Could you check a few things on this model? Use its own coordinates, in mm. Face numbers are marked on the shaded views. A direction names the side the tool comes from. Give positions to 0.01 mm unless a question says otherwise; leave off trailing zeros. Write each loop counter-clockwise with the first axis right and the second up, starting at its lowest first coordinate (ties: lowest second). Pieces come first, ordered by that corner, then holes. Notation, with made-up numbers: (-13.75, 63) - (1.25, 63) arc R20 cw to (1.25, 98) - close; hole circle Ø7 at (87, 20.25). An arc over 180 degrees is marked (long way). Use one line per item in the form item = value.
```python
from build123d import *

# Parameters (mm, degrees)
SKETCH1_W           = 40
SKETCH1_H           = 24
BOSS_EXTRUDE1_DEPTH = 1
SKETCH2_W           = 40
SKETCH2_H           = 24
SKETCH2_W_2         = 21
SKETCH2_H_2         = 17.5
SKETCH2_W_3         = 13
SKETCH2_H_3         = 18.5
BOSS_EXTRUDE3_DEPTH = 8
SKETCH3_W           = 1
SKETCH3_H           = 17.5
CUT_EXTRUDE2_DEPTH  = 3
SKETCH4_W           = 10.24
SKETCH4_H           = 11.92
BOSS_EXTRUDE4_DEPTH = 1.21
CUT_EXTRUDE3_DEPTH  = 2
SKETCH8_W           = 4
SKETCH8_H           = 18.5
CUT_EXTRUDE4_DEPTH  = 5
SKETCH11_W          = 24
SKETCH11_H          = 9
CUT_EXTRUDE5_DEPTH  = 2
SKETCH12_W          = 4
SKETCH12_H          = 3
CUT_EXTRUDE6_DEPTH  = 3
BOSS_EXTRUDE5_DEPTH = 3.5
SKETCH14_W          = 1
SKETCH14_H          = 2.25
CUT_EXTRUDE7_DEPTH  = 3


with BuildPart() as part:
    # Sketch1 → Boss-Extrude1 (new body)
    with BuildSketch(Plane(origin=(0, 0, 0), x_dir=(1, 0, 0), z_dir=(0, 1, 0))):
        with Locations((20, 12)):
            Rectangle(SKETCH1_W, SKETCH1_H)
    extrude(amount=BOSS_EXTRUDE1_DEPTH)

    # Sketch2 → Boss-Extrude3 (add)
    with BuildSketch(Plane(origin=(0, 1, 0), x_dir=(1, 0, 0), z_dir=(0, 1, 0))):
        with Locations((20, 12)):
            Rectangle(SKETCH2_W, SKETCH2_H)
        with Locations((11.5, 12)):
            Rectangle(SKETCH2_W_2, SKETCH2_H_2, mode=Mode.SUBTRACT)
        with Locations((29.5, 12)):
            Rectangle(SKETCH2_W_3, SKETCH2_H_3, mode=Mode.SUBTRACT)
    extrude(amount=BOSS_EXTRUDE3_DEPTH)

    # Sketch3 → Cut-Extrude2 (cut)
    with BuildSketch(Plane(origin=(0, 9, 0), x_dir=(1, 0, 0), z_dir=(0, 1, 0))):
        with Locations((22.5, 12)):
            Rectangle(SKETCH3_W, SKETCH3_H)
    extrude(amount=-CUT_EXTRUDE2_DEPTH, mode=Mode.SUBTRACT)

    # Sketch4 → Boss-Extrude4 (add)
    with BuildSketch(Plane(origin=(0, 1, 0), x_dir=(1, 0, 0), z_dir=(0, 1, 0))):
        with Locations((13.26, 12)):
            Rectangle(SKETCH4_W, SKETCH4_H)
    extrude(amount=BOSS_EXTRUDE4_DEPTH)

    # Sketch5 → Cut-Extrude3 (cut)
    with BuildSketch(Plane(origin=(1, 0, 0), x_dir=(0, 0, -1), z_dir=(1, 0, 0))):
        with BuildLine():
            Line((7.53, 2.25), (7.53, 2.96))
            Line((7.53, 2.96), (7.53, 9))
            Line((7.53, 9), (16.47, 9))
            Line((16.47, 9), (16.47, 2.96))
            Line((16.47, 2.96), (16.47, 2.25))
            ThreePointArc((16.47, 2.25), (16.103883476, 1.366116524), (15.22, 1))
            Line((15.22, 1), (8.78, 1))
            ThreePointArc((8.78, 1), (7.896116524, 1.366116524), (7.53, 2.25))
        make_face()
    extrude(amount=-CUT_EXTRUDE3_DEPTH, mode=Mode.SUBTRACT)

    # Sketch8 → Cut-Extrude4 (cut)
    with BuildSketch(Plane(origin=(0, 9, 0), x_dir=(1, 0, 0), z_dir=(0, 1, 0))):
        with Locations((38, 12)):
            Rectangle(SKETCH8_W, SKETCH8_H)
    extrude(amount=-CUT_EXTRUDE4_DEPTH, mode=Mode.SUBTRACT)

    # Sketch11 → Cut-Extrude5 (cut)
    with BuildSketch(Plane(origin=(40, 0, 0), x_dir=(0, 0, -1), z_dir=(1, 0, 0))):
        with Locations((12, 4.5)):
            Rectangle(SKETCH11_W, SKETCH11_H)
    extrude(amount=-CUT_EXTRUDE5_DEPTH, mode=Mode.SUBTRACT)

    # Sketch12 → Cut-Extrude6 (cut)
    with BuildSketch(Plane(origin=(0, 9, 0), x_dir=(1, 0, 0), z_dir=(0, 1, 0))):
        with Locations((6, 2.5)):
            Rectangle(SKETCH12_W, SKETCH12_H)
    extrude(amount=-CUT_EXTRUDE6_DEPTH, mode=Mode.SUBTRACT)

    # Sketch13 → Boss-Extrude5 (add)
    with BuildSketch(Plane(origin=(0, 9, 0), x_dir=(1, 0, 0), z_dir=(0, 1, 0))):
        Polygon((1, 16.47), (1, 20.75), (3, 20.75), (3, 15.25), (1, 15.25), (1, 16.25), (0, 16.25), (0, 16.47), align=None)
        Polygon((1, 3.25), (3, 3.25), (3, 8.75), (1, 8.75), (1, 7.75), (0, 7.75), (0, 7.53), (1, 7.53), align=None)
    extrude(amount=-BOSS_EXTRUDE5_DEPTH)

    # Sketch14 → Cut-Extrude7 (cut)
    with BuildSketch(Plane(origin=(0, 9, 0), x_dir=(1, 0, 0), z_dir=(0, 1, 0))):
        with Locations((3.5, 2.125)):
            Rectangle(SKETCH14_W, SKETCH14_H)
    extrude(amount=-CUT_EXTRUDE7_DEPTH, mode=Mode.SUBTRACT)


solid = part.part
```
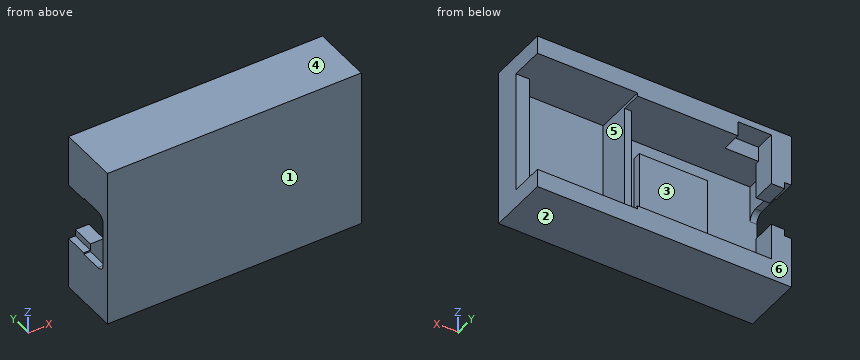
1. Imagine slicing it at C-C, the plane z = -19.25. List the corners of the cut face in (x, y) for me, and give its area (3 significant figures).
Response values:
outline = (0, 0) - (38, 0) - (38, 4) - (36, 4) - (36, 1) - (23, 1) - (23, 6) - (22, 6) - (22, 1) - (1, 1) - (1, 5.5) - (3, 5.5) - (3, 9) - (0, 9) - close
area = 64.0 mm²
2. Imagine slicing it at A-A, the plane y = 8. List the corners of the cut face in (x, z) for me, and give its area (3 significant figures).
Response values:
outline = (0, -24) - (38, -24) - (38, -21.25) - (23, -21.25) - (23, -20.75) - (3, -20.75) - (3, -15.25) - (1, -15.25) - (1, -16.25) - (0, -16.25) - close; (0, -7.75) - (1, -7.75) - (1, -8.75) - (3, -8.75) - (3, -1) - (8, -1) - (8, -3.25) - (23, -3.25) - (23, -2.75) - (38, -2.75) - (38, 0) - (0, 0) - close
area = 252 mm²
3. If we mould it in two halves opening along Z, with no side actions, what happens to the marked faces 1, 2, 3 and 4? For each: pulls with the +Z half, pulls with the -Z half, needs draft (parallel to the pull), parting line crosses it, or undercut.
Response values:
face_1 = needs draft
face_2 = pulls with the -Z half
face_3 = undercut
face_4 = pulls with the +Z half
4. Imagine slicing it at D-D, the plane x = 11.5. List the corners of the cut face in (y, z) for me.
Response values:
outline = (0, -24) - (9, -24) - (9, -20.75) - (1, -20.75) - (1, -17.96) - (2.21, -17.96) - (2.21, -6.04) - (1, -6.04) - (1, -3.25) - (9, -3.25) - (9, 0) - (0, 0) - close
5. Which directions (+Z, -Z, +X, -X, +Y, -Y) give clear straight access to the entire face, cutting with the end or side of a thin tool? Please do the marked faces 5 and 6.
Response values:
face_5 = +Y
face_6 = +Z, -Z, +X, -X, +Y
6. For pin 1 (1.5 mm diameter, centred on x = 1, z = -5.5, fed in from -Y); pin 2 (4 mm diameter, centred on x = 27.5, z = -7.5, fed in from +Y); pin 3 (2 mm diameter, centred on x = 12, z = -14.5, fed in from +Y); pin 4 (2.5 mm diameter, centred on y = 2.5, z = -10.5, fed in from -X), each with a flat end and sliding along its axis, tell me the tip position at first contact or that it passes through.
Response values:
pin_1 = 0
pin_2 = 1
pin_3 = 2.21
pin_4 = 8.14
7. Imagine slicing it at B-B, the plane y = 3.5. List the corners of the cut face in (x, z) for me, and give its area (3 significant figures).
Response values:
outline = (0, -24) - (38, -24) - (38, 0) - (0, 0) - (0, -7.53) - (1, -7.53) - (1, -3.25) - (22, -3.25) - (22, -20.75) - (1, -20.75) - (1, -16.47) - (0, -16.47) - close; hole (23, -21.25) - (36, -21.25) - (36, -2.75) - (23, -2.75) - close
area = 295 mm²
8. If I drill on line 1 (Z direction, x = 17, y = 1.75); line 2 (X direction, y = 3.5, z = -7); line 3 (Z direction, x = 14.5, y = 5.5), over which ranges is the centre line in solid material (lowest first)? Write a range as from..to.
Response values:
line_1 = -24..-20.75, -17.96..-6.04, -3.25..0
line_2 = 0..1, 22..23, 36..38
line_3 = -24..-20.75, -3.25..0
